```python
from build123d import *

# Parameters (mm, degrees)
F4_R   = 22.5
F4_R_2 = 20.5


with BuildPart() as f5:
    # F5: sweep along a path in F0
    with BuildLine(Plane.XZ) as f5_path:
        Line((70.710678, 170.710678), (14.644661, 114.644661))
        ThreePointArc((14.644661, 114.644661), (3.806023, 98.423493), (0, 79.289322))
        Line((0, 79.289322), (0, 0))
    # F4 (on face) → F5 (sweep)
    with BuildSketch(Plane(origin=(120.710678, 0, 120.710678), x_dir=(0, 1, 0), z_dir=(0.707107, 0, 0.707107))):
        with Locations((0, 70.710678)):
            Circle(F4_R)
        with Locations((0, 70.710678)):
            Circle(F4_R_2, mode=Mode.SUBTRACT)
    sweep(path=f5_path.line)


solid = f5.part
```
Work out the finished part from the listing and answer in its coordinate system (mm). Give positions to 0.01 mm unless a question says otherwise; leave off trailing zeros. Write item = value, one per line. Start each with the question number.
(1) The mould has two halves that part along Z. Classify faces 1 (the cylindrical face through (56.658, -2.669, 127.913)), 2 (the flat face through (77.71, -18.23, 163.71)), 3 (the cylindrical face through (55.7, 12.1, 128.87)): +Z half, -Z half, draft (parallel to the pull), parting line (faces both ways), or undercut.
(2) Find the intervals of material crossed by probe 1 along X at (y, z) = (0, 69); probe 2 along X at (y, z) = (15.5, 89); probe 3 along Z at (x, y) = (47, -10.5), in increasing order. Write a range as from..to.
(3) Given pin 1 Ø10 at (x, y) = (69, -7) entering from -Z; pin 2 Ø4 at (x, y) = (6, -3) entering from +Z; pin 3 Ø2 at (y, z) = (6, 120.5) entering from +X, each flat-ended and moving along its own axis, determine where each tip first touches the part or whether it passes through.
From the geometry:
q1.face_1 = undercut
q1.face_2 = +Z half
q1.face_3 = parting line
q2.probe_1 = -22.5..-20.5, 20.5..22.5
q2.probe_2 = -15.59..-12.67, 14.73..17.74
q2.probe_3 = 118.86..122.1, 171.9..175.14
q3.pin_1 = 133.37
q3.pin_2 = 139.57
q3.pin_3 = 52.24
